Design review of the part built by this model. Coordinates are the model's own, in mm. A direction names the side the tool comes from. Give positions to 0.01 mm unless a question says otherwise; leave off trailing zeros. Loops run counter-clockwise (first coordinate to the right, second up) from the corner with the lowest first, then second, coordinate; pieces in that order, holes last. Notation, with made-up numbers: (70, -37) -> (110, -37) arc R18 cw to (110, -24) -> close; hole circle Ø1 at (19.25, -24). An arc over 180 degrees is marked (long way). Use CSV: the item, a comma, the result in double quotes. Start each with the question number.
Item 1: Wall thickness on line 1 along Z through (x, y) = (11.5, 2.45); line 2 along X through (y, z) = (1.3, 2.25); line 3 along X through (y, z) = (1.3, -4): over which ranges is each line inside the solid? List them lowest first. Write a range as from..to.
Item 2: We need section C-C (x = -10). State the section outline as (y, z) points.
Item 3: We need section A-A (y = 1.35). State the section outline as (x, z) points, plus the area to 3 significant figures.
Item 4: For faces 1 (the face through (-7, 2, -4.5)), 2 (the face through (16, 2, 2.5)), 3 (the face through (-17, 2, -2.5)), list the 3-axis set-ups (+Z, -Z, +X, -X, +Y, -Y) from which the entire face can be reached by the end or side of a thin tool; tool diameter is ignored.
Item 5: The part is to be moulded in two halves that separate along X. For faces 4 (the face through (0, 3, 0)), 5 (the face through (2, 2, 3)), 6 (the face through (-15.5, 2, -5)), 7 (the face through (15.5, 2, 5)), say which applies: +X half, -X half, draft (parallel to the pull), parting line (faces both ways), or undercut.
Item 6: Clearance check with flat-ended pins moving along their axes: pin 1 (0.6 mm diameter, centred on x = -17, y = 1, fed in from -Z); pin 2 (1.5 mm diameter, centred on y = 2, z = -5, fed in from -X); pin 3 (0.9 mm diameter, centred on y = 1, z = 5, fed in from +X). State where each tip first meets the part, or that it passes through.
Item 7: We need section B-B (z = 3.75). State the section outline as (x, y) points.
from build123d import *

# Parameters (mm, degrees)
SKETCH1_W           = 35
SKETCH1_H           = 15
BOSS_EXTRUDE1_DEPTH = 3
SKETCH2_W           = 10
SKETCH2_H           = 3
CUT_EXTRUDE1_DEPTH  = 3
SKETCH3_W           = 2
SKETCH3_H           = 5
CUT_EXTRUDE2_DEPTH  = 3


with BuildPart() as part:
    # Sketch1 → Boss-Extrude1 (new body)
    with BuildSketch(Plane(origin=(0, 0, 0), x_dir=(1, 0, 0), z_dir=(0, 1, 0))):
        Rectangle(SKETCH1_W, SKETCH1_H)
    extrude(amount=BOSS_EXTRUDE1_DEPTH)

    # Sketch2 → Cut-Extrude1 (cut)
    with BuildSketch(Plane(origin=(0, 3, 0), x_dir=(1, 0, 0), z_dir=(0, 1, 0))):
        with Locations((-7, -3)):
            Rectangle(SKETCH2_W, SKETCH2_H)
        with Locations((-7, 3)):
            Rectangle(SKETCH2_W, SKETCH2_H)
        with Locations((7, -3)):
            Rectangle(SKETCH2_W, SKETCH2_H)
        with Locations((7, 3)):
            Rectangle(SKETCH2_W, SKETCH2_H)
    extrude(amount=-CUT_EXTRUDE1_DEPTH, mode=Mode.SUBTRACT)

    # Sketch3 → Cut-Extrude2 (cut)
    with BuildSketch(Plane(origin=(0, 3, 0), x_dir=(1, 0, 0), z_dir=(0, 1, 0))):
        with Locations((16.5, 5)):
            Rectangle(SKETCH3_W, SKETCH3_H)
        with Locations((16.5, -5)):
            Rectangle(SKETCH3_W, SKETCH3_H)
        with Locations((-16.5, -5)):
            Rectangle(SKETCH3_W, SKETCH3_H)
        with Locations((-16.5, 5)):
            Rectangle(SKETCH3_W, SKETCH3_H)
    extrude(amount=-CUT_EXTRUDE2_DEPTH, mode=Mode.SUBTRACT)


solid = part.part
Results found:
1,line 1,"-7.5..-4.5, -1.5..1.5, 4.5..7.5"
1,line 2,"-17.5..-12, -2..2, 12..17.5"
1,line 3,"-15.5..-12, -2..2, 12..15.5"
2,outline,"(0, -7.5) -> (3, -7.5) -> (3, -4.5) -> (0, -4.5) -> close; (0, -1.5) -> (3, -1.5) -> (3, 1.5) -> (0, 1.5) -> close; (0, 4.5) -> (3, 4.5) -> (3, 7.5) -> (0, 7.5) -> close"
3,outline,"(-17.5, -2.5) -> (-15.5, -2.5) -> (-15.5, -7.5) -> (15.5, -7.5) -> (15.5, -2.5) -> (17.5, -2.5) -> (17.5, 2.5) -> (15.5, 2.5) -> (15.5, 7.5) -> (-15.5, 7.5) -> (-15.5, 2.5) -> (-17.5, 2.5) -> close; hole (-12, -4.5) -> (-2, -4.5) -> (-2, -1.5) -> (-12, -1.5) -> close; hole (-12, 1.5) -> (-2, 1.5) -> (-2, 4.5) -> (-12, 4.5) -> close; hole (2, -4.5) -> (12, -4.5) -> (12, -1.5) -> (2, -1.5) -> close; hole (2, 1.5) -> (12, 1.5) -> (12, 4.5) -> (2, 4.5) -> close"
3,area,"365 mm²"
4,face 1,"+Y, -Y"
4,face 2,"+Z, +X, +Y, -Y"
4,face 3,"-Z, -X, +Y, -Y"
5,face 4,"draft"
5,face 5,"undercut"
5,face 6,"-X half"
5,face 7,"+X half"
6,pin 1,"z = -2.5"
6,pin 2,"x = -15.5"
6,pin 3,"x = 15.5"
7,outline,"(-15.5, 0) -> (-12, 0) -> (-12, 3) -> (-15.5, 3) -> close; (-2, 0) -> (2, 0) -> (2, 3) -> (-2, 3) -> close; (12, 0) -> (15.5, 0) -> (15.5, 3) -> (12, 3) -> close"
